```python
from build123d import *

# Parameters (mm, degrees)
F0_W          = 62
F0_H          = 23
F1_DEPTH      = 75
F1_DEPTH_BACK = 75
F2_R          = 9
F3_R          = 5
F4_W          = 13
F4_H          = 5
F5_DEPTH      = 10


with BuildPart() as f1:
    # F0 (on Front) → F1 (new body, two sides)
    with BuildSketch(Plane.XZ) as f1_sk:
        Rectangle(F0_W, F0_H)
    extrude(amount=F1_DEPTH)
    extrude(f1_sk.sketch, amount=-F1_DEPTH_BACK)

    # F2
    f2_edges = [f1.edges().sort_by_distance(p)[0] for p in [
        (31, 0, 11.5),
        (31, 0, -11.5),
        (-31, 0, 11.5),
        (-31, 0, -11.5),
    ]]
    fillet(f2_edges, radius=F2_R)

    # F3
    f3_edges = [f1.edges().sort_by_distance(p)[0] for p in [
        (0, -75, -11.5),
        (-28.363961, -75, -8.863961),
        (28.363961, -75, -8.863961),
        (-31, -75, 0),
        (31, -75, 0),
        (-28.363961, -75, 8.863961),
        (28.363961, -75, 8.863961),
        (0, -75, 11.5),
        (0, 75, -11.5),
        (-28.363961, 75, -8.863961),
        (28.363961, 75, -8.863961),
        (-31, 75, 0),
        (31, 75, 0),
        (-28.363961, 75, 8.863961),
        (28.363961, 75, 8.863961),
        (0, 75, 11.5),
    ]]
    fillet(f3_edges, radius=F3_R)

    # F4 (on face) → F5 (cut)
    with BuildSketch(Plane.XZ.offset(75)):
        with Locations((-16.5, 0)):
            Rectangle(F4_W, F4_H)
        with Locations((16.5, 0)):
            Rectangle(F4_W, F4_H)
    extrude(amount=-F5_DEPTH, mode=Mode.SUBTRACT)


solid = f1.part
```
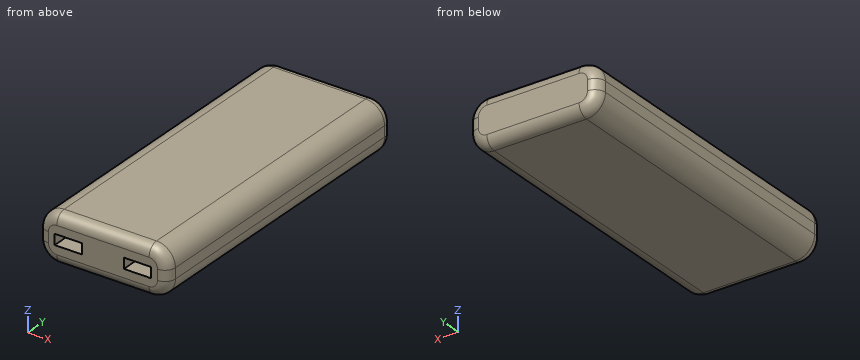
Can you work these out from the model? Positions are in its coordinate system, mm. Give positions to 0.01 mm unless a question says otherwise; leave off trailing zeros. Order: outer loops, then holes, each group sorted by start corner. A loop starts at its lowest first (then second) coordinate and runs counter-clockwise, first axis right, second up. Notation, with made-up numbers: (43, -17.5) - (59, -17.5) arc R10 cw to (59, -7.5) - close; hole circle Ø2 at (87.25, -24). An arc over 180 degrees is marked (long way). Use a Markdown table: item, result. Add a question column.
Q1. If we section it at B-B on x = -12.5: Write out the boundary of the cut face in (y, z).
Q2. Please list where these lines run through material, in increasing order: line 1 along Z through (x, y) = (22.5, 27.5); line 2 along X through (y, z) = (64, 7.75); line 3 along X through (y, z) = (46, 8.5).
Q3. If we section it at C-C on z = -1: Write out the boundary of the cut face in (x, y).
Q4. If we section it at A-A on y = 6.5: Write out the boundary of the cut face in (x, z), plus the area to 3 significant figures.
Q5. I'm going to push flat-ended pins straight in: pin 1 (2.5 mm diameter, centred on x = 18, z = -1, fed in from -Y); pin 2 (1.5 mm diameter, centred on y = -71, z = 0.5, fed in from +X). Where does each tip first touch, or does it pass through?
Answers follow:
| question | item | result |
|---|---|---|
| 1 | outline | (-75, -6.5) arc R5 ccw to (-70, -11.5) - (70, -11.5) arc R5 ccw to (75, -6.5) - (75, 6.5) arc R5 ccw to (70, 11.5) - (-70, 11.5) arc R5 ccw to (-75, 6.5) - (-75, 2.5) - (-65, 2.5) - (-65, -2.5) - (-75, -2.5) - close |
| 2 | line 1 | z = -11.49 to 11.49 |
| 2 | line 2 | x = -29.31 to 29.31 |
| 2 | line 3 | x = -28.71 to 28.71 |
| 3 | outline | (-31, -70) arc R5 ccw to (-26, -75) - (-23, -75) - (-23, -65) - (-10, -65) - (-10, -75) - (10, -75) - (10, -65) - (23, -65) - (23, -75) - (26, -75) arc R5 ccw to (31, -70) - (31, 70) arc R5 ccw to (26, 75) - (-26, 75) arc R5 ccw to (-31, 70) - close |
| 4 | outline | (-31, -2.5) arc R9 ccw to (-22, -11.5) - (22, -11.5) arc R9 ccw to (31, -2.5) - (31, 2.5) arc R9 ccw to (22, 11.5) - (-22, 11.5) arc R9 ccw to (-31, 2.5) - close |
| 4 | area | 1,360 mm^2 |
| 5 | pin 1 | stops at y = -65 |
| 5 | pin 2 | stops at x = 30.99 |
